Verification items for the finished model (mm, model axes). A direction names the side the tool comes from. Give positions to 0.01 mm unless a question says otherwise; leave off trailing zeros. Write each loop counter-clockwise with the first axis right and the second up, starting at its lowest first coordinate (ties: lowest second). Pieces come first, ordered by that corner, then holes. Notation, with made-up numbers: (57.5, 5.25) - (97.5, 5.25) arc R17 cw to (97.5, 14.25) - close; hole circle Ø2 at (-26.5, 56). An arc over 180 degrees is marked (long way). Put each result on its own line as item: value.
Autodesk Fusion 360 part; units mm, degrees
sketch "スケッチ1" plane through (0, 0, 0) normal (0, 0, 1) x (1, 0, 0)
  line L0 (0, 100) -> (0, -100)
  line L1 (200, -100) -> (200, 100)
  line L2 (188, -17) -> (188, -100)
  line L3 (12, -100) -> (12, -17)
  line L4 (0, -100) -> (12, -100)
  line L5 (188, -100) -> (200, -100)
  line L6 (12, 17) -> (12, 100)
  line L7 (188, 100) -> (188, 17)
  line L8 (175, 4) -> (25, 4)
  line L9 (25, -4) -> (175, -4)
  arc A0 (25, -4) -> (12, -17) centre (25, -17) ccw
  arc A1 (12, 17) -> (25, 4) centre (25, 17) ccw
  arc A2 (188, -17) -> (175, -4) centre (175, -17) ccw
  arc A3 (175, 4) -> (188, 17) centre (175, 17) ccw
  line L10 (12, 100) -> (0, 100)
  line L11 (200, 100) -> (188, 100)
extrude "押し出し1" add sketch "スケッチ1" along normal blind 100
Q1. Go/stop test with flat-tipped pins: pin 1 Ø4 at (x, z) = (155.5, 46) entering from -Y; pin 2 Ø2 at (x, z) = (165, 41.5) entering from +Y. Record where each tip stops, or that it passes through.
Answers follow:
pin 1: stops at y = -4
pin 2: stops at y = 4
Q2. Scan lines: line 1 along X through (y, z) = (46, 44); line 2 along Y through (x, z) = (68, 67.5); line 3 along Y through (x, z) = (16.5, 75). Record each from-to range of solid material in increasing order.
Answers follow:
line 1: x = 0 to 12, 188 to 200
line 2: y = -4 to 4
line 3: y = -7.16 to 7.16
Q3. Section check B-B, the plane z = 49.5. Record the cut outline in (x, y), plus the area to 3 significant figures.
Answers follow:
outline: (0, -100) - (12, -100) - (12, -17) arc R13 cw to (25, -4) - (175, -4) arc R13 cw to (188, -17) - (188, -100) - (200, -100) - (200, 100) - (188, 100) - (188, 17) arc R13 cw to (175, 4) - (25, 4) arc R13 cw to (12, 17) - (12, 100) - (0, 100) - close
area: 6,350 mm2
Q4. Set-up check for faces 1 (the face through (184.293, 7.909, 49.3)), 2 (the face through (99, -4, 49)), 3 (the face through (6, 100, 49)): record each of +Z, -Z, +X, -X, +Y, -Y from which the full face is reachable in a straight line by a thin tool's end or side.
Answers follow:
face 1: +Z, -Z, +Y
face 2: +Z, -Z, -Y
face 3: +Z, -Z, +X, -X, +Y
Q5. Section check C-C, the plane x = 147.5. Record the cut outline in (y, z), plus the area to 3 significant figures.
Answers follow:
outline: (-4, 0) - (4, 0) - (4, 100) - (-4, 100) - close
area: 800 mm2
Q6. Release check for a two-part mould opening along X. For faces 4 (the face through (100, 0, 0)), 5 (the face through (188, 59, 49)), 6 (the face through (200, -1, 49)), 7 (the face through (101, 4, 49)) record: released by +X, released by -X, zero draft, split by the parting line, or undercut.
Answers follow:
face 4: zero draft
face 5: undercut
face 6: released by +X
face 7: undercut
Q7. Section check A-A, the plane y = 20.5. Record the cut outline in (x, z), plus the area to 3 significant figures.
Answers follow:
outline: (0, 0) - (12, 0) - (12, 100) - (0, 100) - close; (188, 0) - (200, 0) - (200, 100) - (188, 100) - close
area: 2,400 mm2
